```python
from build123d import *

# Parameters (mm, degrees)
ESQUISSE1_W      = 60
ESQUISSE1_H      = 70
EXTRUSION1_DEPTH = 10
EXTRUSION2_REACH = 53.55
ESQUISSE2_R      = 0.5
ESQUISSE4_W      = 25
ESQUISSE4_H      = 10
EXTRUSION3_DEPTH = 60
EXTRUSION4_DEPTH = 60


with BuildPart() as part:
    # Esquisse1 → Extrusion1 (new body)
    with BuildSketch(Plane.XY):
        with Locations((-4.316825769, -2.145652174)):
            Rectangle(ESQUISSE1_W, ESQUISSE1_H)
    extrude(amount=EXTRUSION1_DEPTH)

    # Esquisse2 → Extrusion2 (cut, up to next)
    with BuildSketch(Plane(origin=(0, 0, 0), x_dir=(-1, 0, 0), z_dir=(0, 0, -1)), mode=Mode.PRIVATE) as extrusion2_sk1:
        with Locations((4.316825769, 2.854347826)):
            Circle(ESQUISSE2_R)
    extrusion2_tool1 = extrude(extrusion2_sk1.sketch, amount=-EXTRUSION2_REACH, mode=Mode.PRIVATE) & part.part
    add(extrusion2_tool1.solids().sort_by_distance((-4.316826, 2.854348, 0))[0], mode=Mode.SUBTRACT)

    # Esquisse4 → Extrusion3 (add)
    with BuildSketch(Plane(origin=(0, 32.854347826, 0), x_dir=(1, 0, 0), z_dir=(0, 1, 0))):
        with Locations((-21.816825769, -5)):
            Rectangle(ESQUISSE4_W, ESQUISSE4_H)
    extrude(amount=EXTRUSION3_DEPTH)

    # Esquisse5 → Extrusion4 (add)
    with BuildSketch(Plane(origin=(0, 0, 0), x_dir=(-1, 0, 0), z_dir=(0, 0, -1))):
        Polygon((29.316825769, 25.271005401), (24.959851341, 12.996610653), (29.400349472, 11.420391442), (34.316825769, 25.271005401), (34.316825769, 92.854347826), (29.316825769, 92.854347826), align=None)
        Polygon((9.316825769, 92.854347826), (14.316825769, 92.854347826), (14.316825769, 23.566663003), (9.316825769, 25.271005401), align=None)
    extrude(amount=EXTRUSION4_DEPTH)


solid = part.part
```
Verification items for the finished model (mm, model axes). A direction names the side the tool comes from. Give positions to 0.01 mm unless a question says otherwise; leave off trailing zeros. Order: outer loops, then holes, each group sorted by start corner. A loop starts at its lowest first (then second) coordinate and runs counter-clockwise, first axis right, second up. Notation, with made-up numbers: (35, 34.25) - (55, 34.25) arc R21 ccw to (55, 68.25) - close; hole circle Ø7 at (40, 40). An arc over 180 degrees is marked (long way). Answer as CSV lines item,"result". Start each with the question number.
Item 1: Section check C-C, the plane z = 4. Record the boundary of the cut face in (x, y), plus the area to 3 significant figures.
Item 2: Material ranges on L1, parallel to X at y = 45, z = -38; L2, parallel to Z at x = -22.5, y = 29; L3, parallel to Y at x = 19, z = 6.5, recorded low to high.
Item 3: Gauge pin test, flat ends, axial feed: pin 1 (10 mm diameter, centred on x = -16, y = 3.5, fed in from -Z); pin 2 (10 mm diameter, centred on y = 8, z = -49, fed in from -X); pin 3 (8 mm diameter, centred on x = 8.5, z = 2.5, fed in from +Y). Record the tip position at first contact, or that the pin passes through.
Item 4: Section check D-D, the plane x = 11. Record the boundary of the cut face in (y, z), plus the area to 3 significant figures.
Item 5: Section check B-B, the plane y = 28. Record the boundary of the cut face in (x, z), plus the area to 3 significant figures.
Item 6: Section check A-A, the plane z = -32. Record the boundary of the cut face in (x, y), plus the area to 3 significant figures.
Item 7: Mould release check, pull along X, two halves, no side actions. Record for faces 5 (the face through (8, 32.854, 5)), 6 (the face through (-34.317, 56, -25)), 7 (the face through (-29.317, 60, -30)): released by +X, released by -X, zero draft, split by the parting line, or undercut.
Item 8: Access from +Z, -Z, +X, -X, +Y, -Y to the whole of each face (thin tool, end or side, straight path). Record for faces 1 (the face through (25.683, -3, 5)), 2 (the face through (-27.15, 12.22, -29.58)), 3 (the face through (-31.824, 18.249, -29.58)), 4 (the face through (-14.317, 59, -30)).
Filled in:
1,outline,"(-34.32, -37.15) - (25.68, -37.15) - (25.68, 32.85) - (-9.32, 32.85) - (-9.32, 92.85) - (-34.32, 92.85) - close; hole circle Ø1 at (-4.32, 2.85)"
1,area,"5,700 mm^2"
2,L1,"-34.32 to -29.32, -14.32 to -9.32"
2,L2,"0 to 10"
2,L3,"-37.15 to 32.85"
3,pin 1,"z = 0"
3,pin 2,"x = -29.96"
3,pin 3,"y = 32.85"
4,outline,"(-37.15, 0) - (32.85, 0) - (32.85, 10) - (-37.15, 10) - close"
4,area,"700 mm^2"
5,outline,"(-34.32, -60) - (-29.32, -60) - (-29.32, 0) - (-14.32, 0) - (-14.32, -60) - (-9.32, -60) - (-9.32, 0) - (25.68, 0) - (25.68, 10) - (-34.32, 10) - close"
5,area,"1,200 mm^2"
6,outline,"(-34.32, 25.27) - (-29.4, 11.42) - (-24.96, 13) - (-29.32, 25.27) - (-29.32, 92.85) - (-34.32, 92.85) - close; (-14.32, 23.57) - (-9.32, 25.27) - (-9.32, 92.85) - (-14.32, 92.85) - close"
6,area,"745 mm^2"
7,face 5,"zero draft"
7,face 6,"released by -X"
7,face 7,"undercut"
8,face 1,"+Z, -Z, +X, +Y, -Y"
8,face 2,"-Z, +X, -Y"
8,face 3,"-Z, -X, -Y"
8,face 4,"-Z, +Y, -Y"
